Part model, mm, in its own coordinate system. Coordinates: 2 decimals unless noted, no trailing zeros. Order: outer loops, then holes, each group sorted by start corner. A loop starts at its lowest first (then second) coordinate and runs counter-clockwise, first axis right, second up.
1) Cut at A-A (z = 0). List the corners of the cut face in (x, y), and give its area (3 significant figures).
2) Pin check, flat tips, straight feed: pin 1 Ø1.5 at (x, y) = (2.5, 6.5) entering from +Z; pin 2 Ø1.5 at (y, z) = (16.5, 2) entering from -X; pin 3 Ø1.5 at (x, y) = (-1.5, 10) entering from +Z. Stop position of each tip, or through.
3) Cut at B-B (x = -2.5). List the corners of the cut face in (y, z).
4) Cut at D-D (y = 12.25). List the corners of the cut face in (x, z).
5) Wall check: L1, parallel to Y at x = 0, z = 4.6; L2, parallel to Z at x = 0, y = 12.5; L3, parallel to X at y = 8.75, z = 1.5. Give the ranges that are in metal, low to high.
6) Mould opens along Y. For faces 1 (the flat face through (4, 0, -2)), 2 (the flat face through (4, 25, -2)), 3 (the cylindrical face through (1.57, 5.35, -4.6)), 4 (the cylindrical face through (1.57, 18.35, -4.6)) say: +Y half, -Y half, draft (parallel to the pull), parting line (faces both ways), or undercut.
7) Cut at C-C (x = 0). List the corners of the cut face in (y, z), and give its area (3 significant figures).
Autodesk Inventor part; units mm, degrees
ref_plane "YZ Plane" through (0, 0, 0) normal (1, 0, 0) x (0, 1, 0)
ref_plane "XZ Plane" through (0, 0, 0) normal (0, 1, 0) x (-1, 0, 0)
ref_plane "XY Plane" through (0, 0, 0) normal (0, 0, 1) x (1, 0, 0)
sketch "Sketch1" plane through (0, 0, 0) normal (0, 1, 0) x (-1, 0, 0)
  circle A0 centre (0, 0) radius 5.55
  circle A1 centre (0, 0) radius 4.05
  dimension "d0" = 11.1
  dimension "d1" = 8.1
extrude "Extrusion1" add sketch "Sketch1" along normal blind 25
sketch "Sketch2" plane through (0, 0, 0) normal (0, 0, 1) x (1, 0, 0)
  line L0 (5.55, 25) -> (-5.55, 25)
  line L1 (5.55, 0) -> (-5.55, 0)
  circle A0 centre (0, 6) radius 1.7
  line L2 (5.55, 0) -> (-5.55, 0)
  line L3 (-4.05, 25) -> (-4.05, 0)
  circle A1 centre (0, 19) radius 1.7
  point P0 (0, 0)
  point P1 (0, 25)
  dimension "d4" = 3.4
  dimension "d5" = 6
  dimension "d6" = 3.4
  dimension "d7" = 6
extrude "Extrusion2" cut sketch "Sketch2" along normal mid plane 25
properties part number "ACOMPLE_PLASTICO" material "Steel, Mild, Welded"
Geometry check:
1. outline: (-5.55, 0) - (-4.05, 0) - (-4.05, 25) - (-5.55, 25) - close; (4.05, 0) - (5.55, 0) - (5.55, 25) - (4.05, 25) - close
1. area: 75.0 mm2
2. pin 1: stops at z = 5.27
2. pin 2: stops at x = -5.41
2. pin 3: stops at z = 5.5
3. outline: (0, -4.96) - (25, -4.96) - (25, -3.19) - (0, -3.19) - close; (0, 3.19) - (25, 3.19) - (25, 4.96) - (0, 4.96) - close
4. outline: circle Ø11.1 at (0, 0); hole circle Ø8.1 at (0, 0)
5. L1: y = 0 to 4.3, 7.7 to 17.3, 20.7 to 25
5. L2: z = -5.55 to -4.05, 4.05 to 5.55
5. L3: x = -5.34 to -3.76, 3.76 to 5.34
6. face 1: -Y half
6. face 2: +Y half
6. face 3: undercut
6. face 4: undercut
7. outline: (0, -5.55) - (4.3, -5.55) - (4.3, -4.05) - (0, -4.05) - close; (0, 4.05) - (4.3, 4.05) - (4.3, 5.55) - (0, 5.55) - close; (7.7, -5.55) - (17.3, -5.55) - (17.3, -4.05) - (7.7, -4.05) - close; (7.7, 4.05) - (17.3, 4.05) - (17.3, 5.55) - (7.7, 5.55) - close; (20.7, -5.55) - (25, -5.55) - (25, -4.05) - (20.7, -4.05) - close; (20.7, 4.05) - (25, 4.05) - (25, 5.55) - (20.7, 5.55) - close
7. area: 54.6 mm2
